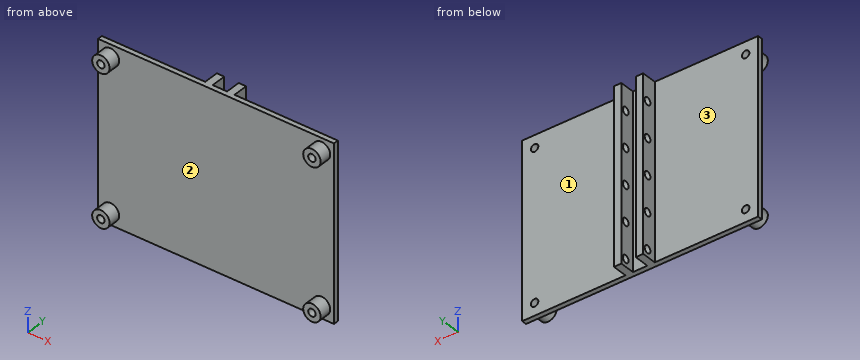
from build123d import *

# Parameters (mm, degrees)
SKETCH_1_W          = 95
SKETCH_1_H          = 70
SKETCH_1_R          = 1.5
EXTRUDE_1_DEPTH     = 2
SKETCH_2_W          = 3
SKETCH_2_H          = 70
EXTRUDE_2_DEPTH     = 6
SKETCH_3_R          = 1.5
CUT_EXTRUDE_1_DEPTH = 54.4
SKETCH_4_R          = 3.5
SKETCH_4_R_2        = 1.5
EXTRUDE_3_DEPTH     = 5


with BuildPart() as part:
    # 草图1 → 凸台-拉伸1 (new body)
    with BuildSketch(Plane(origin=(0, 0, 0), x_dir=(1, 0, 0), z_dir=(0, 1, 0))):
        Rectangle(SKETCH_1_W, SKETCH_1_H)
        with Locations((-42.5, 30)):
            Circle(SKETCH_1_R, mode=Mode.SUBTRACT)
        with Locations((42.5, 30)):
            Circle(SKETCH_1_R, mode=Mode.SUBTRACT)
        with Locations((-42.5, -30)):
            Circle(SKETCH_1_R, mode=Mode.SUBTRACT)
        with Locations((42.5, -30)):
            Circle(SKETCH_1_R, mode=Mode.SUBTRACT)
    extrude(amount=EXTRUDE_1_DEPTH)

    # 草图2 → 凸台-拉伸2 (add)
    with BuildSketch(Plane(origin=(0, 2, 0), x_dir=(1, 0, 0), z_dir=(0, 1, 0))):
        with Locations((-4.4, 0)):
            Rectangle(SKETCH_2_W, SKETCH_2_H)
        with Locations((4.4, 0)):
            Rectangle(SKETCH_2_W, SKETCH_2_H)
    extrude(amount=EXTRUDE_2_DEPTH)

    # 草图3 → 切除-拉伸1 (cut, through all)
    with BuildSketch(Plane.ZY.offset(5.9)):
        with Locations((-31.985850954, 5.75)):
            Circle(SKETCH_3_R)
        with Locations((-17.635850954, 5.75)):
            Circle(SKETCH_3_R)
        with Locations((-3.285850954, 5.75)):
            Circle(SKETCH_3_R)
        with Locations((11.064149046, 5.75)):
            Circle(SKETCH_3_R)
        with Locations((25.414149046, 5.75)):
            Circle(SKETCH_3_R)
    extrude(amount=-CUT_EXTRUDE_1_DEPTH, mode=Mode.SUBTRACT)

    # 草图4 → 凸台-拉伸3 (add)
    with BuildSketch(Plane.XZ):
        with Locations((-42.5, -30)):
            Circle(SKETCH_4_R)
        with Locations((-42.5, -30)):
            Circle(SKETCH_4_R_2, mode=Mode.SUBTRACT)
        with Locations((-42.5, 30)):
            Circle(SKETCH_4_R)
        with Locations((-42.5, 30)):
            Circle(SKETCH_4_R_2, mode=Mode.SUBTRACT)
        with Locations((42.5, 30)):
            Circle(SKETCH_4_R)
        with Locations((42.5, 30)):
            Circle(SKETCH_4_R_2, mode=Mode.SUBTRACT)
        with Locations((42.5, -30)):
            Circle(SKETCH_4_R)
        with Locations((42.5, -30)):
            Circle(SKETCH_4_R_2, mode=Mode.SUBTRACT)
    extrude(amount=EXTRUDE_3_DEPTH)


solid = part.part
Read the model definition and answer for the solid it produces. Units are mm, in the model's axes. Face numbers are marked on the shaded views. A direction names the side the tool comes from. Give positions to 0.01 mm unless a question says otherwise; leave off trailing zeros. Write each loop counter-clockwise with the first axis right and the second up, starting at its lowest first coordinate (ties: lowest second). Pieces come first, ordered by that corner, then holes. Notation, with made-up numbers: (68.5, 55) - (101.5, 55) arc R9 ccw to (101.5, 63) - close; hole circle Ø6 at (3, -26.5). An arc over 180 degrees is marked (long way). Use CSV: the item, a comma, the result in double quotes. Start each with the question number.
(1) Find section D-D (y = 5.75). Count the separate pieces of the cut face and the enclosed holes in it, plus the area to 3 significant figures.
(2) For the marked faces 1, 2 and 3, determine the directions among +Z, -Z, +X, -X, +Y, -Y from which every point of the face is accessible in a straight line to the end or side of a thin tool.
(3) Find section B-B (z = 30). Give the vertices of the cut face in (x, y).
(4) Consider line 1 along X through (y, z) = (7.75, 30); line 2 along Y through (x, z) = (24.5, -15.5); line 3 along Z through (x, y) = (40.5, -2.5). Determine where each line is inside the solid, lowest interval first.
(5) Find section A-A (y = -2). Give the vertices of the cut face in (x, z).
(6) Given P1, Ø8, axis at x = 15.5, z = -8.5, coming from the -Y side; P2, Ø2.5, axis at y = 5.75, z = 25.41, coming from the -X side; P3, Ø3.5, axis at y = 5.75, z = -3.29, coming from the +X side; P4, Ø1.8, axis at y = 4, z = 7.5, coming from the -X side, each flat-ended and moving along its own axis, determine where each tip first touches the part or whether it passes through.
(7) Find section C-C (x = 42.5). Give the vertices of the cut face in (y, z), plus the area to 3 significant figures.
Findings below:
1,separate pieces,"12"
1,enclosed holes,"0"
1,area,"330 mm2"
2,face 1,"+Z, -Z, +X, +Y"
2,face 2,"-Y"
2,face 3,"+Z, -Z, -X, +Y"
3,outline,"(-47.5, 0) - (-46, 0) - (-46, -5) - (-44, -5) - (-44, 2) - (-47.5, 2) - close; (-41, -5) - (-39, -5) - (-39, 0) - (39, 0) - (39, -5) - (41, -5) - (41, 2) - (5.9, 2) - (5.9, 8) - (2.9, 8) - (2.9, 2) - (-2.9, 2) - (-2.9, 8) - (-5.9, 8) - (-5.9, 2) - (-41, 2) - close; (44, -5) - (46, -5) - (46, 0) - (47.5, 0) - (47.5, 2) - (44, 2) - close"
4,line 1,"-5.9 to -2.9, 2.9 to 5.9"
4,line 2,"0 to 2"
4,line 3,"-32.87 to -27.13, 27.13 to 32.87"
5,outline,"circle Ø7 at (-42.5, -30); circle Ø7 at (-42.5, 30); circle Ø7 at (42.5, -30); circle Ø7 at (42.5, 30); hole circle Ø3 at (-42.5, -30); hole circle Ø3 at (-42.5, 30); hole circle Ø3 at (42.5, -30); hole circle Ø3 at (42.5, 30)"
6,P1,"y = 0"
6,P2,"through"
6,P3,"x = 5.9"
6,P4,"x = -5.9"
7,outline,"(-5, -33.5) - (0, -33.5) - (0, -35) - (2, -35) - (2, -31.5) - (-5, -31.5) - close; (-5, -28.5) - (2, -28.5) - (2, 28.5) - (-5, 28.5) - (-5, 26.5) - (0, 26.5) - (0, -26.5) - (-5, -26.5) - close; (-5, 31.5) - (2, 31.5) - (2, 35) - (0, 35) - (0, 33.5) - (-5, 33.5) - close"
7,area,"168 mm2"
